Can you work these out from the model? Positions are in its coordinate system, mm. Face numbers are marked on the shaded views. Round coordinates to 2 decimals unless told otherwise and drop trailing zeros. Order: outer loops, then holes, each group sorted by start corner. A loop starts at its lowest first (then second) coordinate and runs counter-clockwise, first axis right, second up. Notation, with made-up numbers: (-11, 47.5) -> (3, 47.5) arc R31 cw to (3, 73.5) -> close; hole circle Ø8 at (30.25, 79). An arc over 180 degrees is marked (long way). One line per item, written item: value.
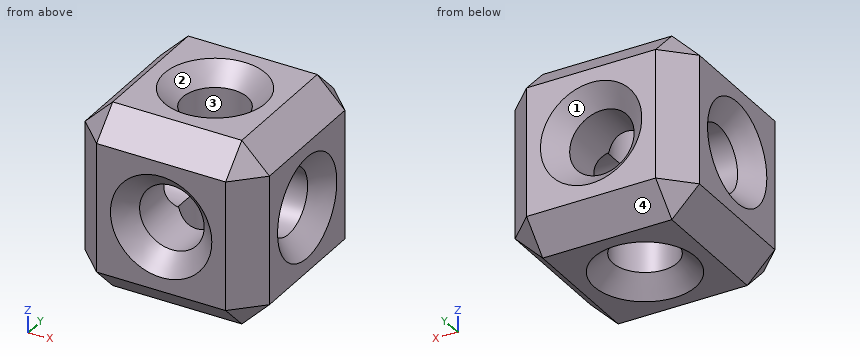
```python
from build123d import *

# Parameters (mm, degrees)
F0_W     = 100
F0_H     = 100
F0_R     = 17.5
F1_DEPTH = 50
F2_R     = 17.5
F3_DEPTH = 100
F4_R     = 17.5
F5_DEPTH = 100
F6_SIZE  = 15
F7_SIZE  = 10


with BuildPart() as f1:
    # F0 (on Front) → F1 (new body, symmetric)
    with BuildSketch(Plane.XZ):
        Rectangle(F0_W, F0_H)
        Circle(F0_R, mode=Mode.SUBTRACT)
    extrude(amount=F1_DEPTH, both=True)

    # F2 (on face) → F3 (cut, through all)
    with BuildSketch(Plane(origin=(-50, 0, 0), x_dir=(0, -1, 0), z_dir=(-1, 0, 0))):
        Circle(F2_R)
    extrude(amount=-F3_DEPTH, mode=Mode.SUBTRACT)

    # F4 (on face) → F5 (cut, through all)
    with BuildSketch(Plane(origin=(0, 0, -50), x_dir=(1, 0, 0), z_dir=(0, 0, -1))):
        Circle(F4_R)
    extrude(amount=-F5_DEPTH, mode=Mode.SUBTRACT)

    # F6
    f6_edges = [f1.edges().sort_by_distance(p)[0] for p in [
        (0, 50, 50),
        (50, 0, 50),
        (0, -50, 50),
        (-50, 0, 50),
        (-50, 50, 0),
        (-50, -50, 0),
        (-50, 0, -50),
        (0, 50, -50),
        (50, 0, -50),
        (50, -50, 0),
        (0, -50, -50),
        (50, 50, 0),
    ]]
    chamfer(f6_edges, length=F6_SIZE)

    # F7
    f7_edges = [f1.edges().sort_by_distance(p)[0] for p in [
        (50, 17.5, 0),
        (-17.5, 50, 0),
        (-17.5, 0, -50),
        (-17.5, -50, 0),
        (-50, 17.5, 0),
        (-17.5, 0, 50),
    ]]
    chamfer(f7_edges, length=F7_SIZE)


solid = f1.part
```
Q1. I want a section at A-A on y = 0. List the corners of the cut face in (x, z) for me, plus the area to 4 significant figures.
Answers below:
outline: (-50, -35) -> (-35, -50) -> (-27.5, -50) -> (-17.5, -40) -> (-17.5, -17.5) -> (-40, -17.5) -> (-50, -27.5) -> close; (-50, 27.5) -> (-40, 17.5) -> (-17.5, 17.5) -> (-17.5, 40) -> (-27.5, 50) -> (-35, 50) -> (-50, 35) -> close; (17.5, -40) -> (27.5, -50) -> (35, -50) -> (50, -35) -> (50, -27.5) -> (40, -17.5) -> (17.5, -17.5) -> close; (17.5, 17.5) -> (40, 17.5) -> (50, 27.5) -> (50, 35) -> (35, 50) -> (27.5, 50) -> (17.5, 40) -> close
area: 3,375 mm^2
Q2. I want a section at D-D on z = 37.5. List the corners of the cut face in (x, y) for me.
Answers below:
outline: (-47.5, -35) -> (-35, -47.5) -> (35, -47.5) -> (47.5, -35) -> (47.5, 35) -> (35, 47.5) -> (-35, 47.5) -> (-47.5, 35) -> close; hole circle Ø35 at (0, 0)
Q3. I want a section at C-C on x = -32. List the corners of the cut face in (y, z) for me.
Answers below:
outline: (-50, -35) -> (-35, -50) -> (35, -50) -> (50, -35) -> (50, 35) -> (35, 50) -> (-35, 50) -> (-50, 35) -> close; hole circle Ø35 at (0, 0)
Q4. We'd pull the mould along Z, two halves only. Please class the marked faces 1, 2, 3 and 4: released by +Z, released by -Z, zero draft, split by the parting line, or undercut.
Answers below:
face 1: undercut
face 2: released by +Z
face 3: zero draft
face 4: released by -Z
Q5. Will these pins go through, and if not, where does the flat tip stop? pin 1 Ø3 at (x, y) = (-17, -10) entering from -Z; pin 2 Ø6 at (x, y) = (20, -6.5) entering from +Z; pin 3 Ø1.5 at (x, z) = (39.5, 36.5) entering from -Y.
Answers below:
pin 1: z = -43.72
pin 2: z = 46.53
pin 3: y = -45.06
Q6. Please list where these lines run through material, in increasing order: line 1 along Z through (x, y) = (-31, 0); line 2 along Y through (x, z) = (-4, -22).
Answers below:
line 1: -50 to -17.5, 17.5 to 50
line 2: -44.86 to -17.04, 17.04 to 44.86
